Autodesk Inventor part; units mm, degrees
ref_plane "YZ Plane" through (0, 0, 0) normal (1, 0, 0) x (0, 1, 0)
ref_plane "XZ Plane" through (0, 0, 0) normal (0, 1, 0) x (-1, 0, 0)
ref_plane "XY Plane" through (0, 0, 0) normal (0, 0, 1) x (1, 0, 0)
sketch "スケッチ1" plane through (0, 0, 0) normal (0, 0, 1) x (1, 0, 0)
  line L0 (-4.5, 75) -> (4.5, 75)
  line L1 (4.5, 75) -> (4.5, -75)
  line L2 (4.5, -75) -> (-4.5, -75)
  line L3 (-4.5, -75) -> (-4.5, 75)
  line L4 (-4.5, 75) -> (4.5, -75) construction
  line L5 (4.5, 75) -> (-4.5, -75) construction
  circle A0 centre (0, 70) radius 1.7
  circle A1 centre (0, 50) radius 1.7
  circle A2 centre (0, 30) radius 1.7
  circle A3 centre (0, 10) radius 1.7
  circle A4 centre (0, -10) radius 1.7
  circle A5 centre (0, -30) radius 1.7
  circle A6 centre (0, -50) radius 1.7
  circle A7 centre (0, -70) radius 1.7
  point P0 (0, 0)
  dimension "d0" = 9
  dimension "d1" = 150
  dimension "d2" = 3.4
  dimension "d3" = 3.4
  dimension "d4" = 3.4
  dimension "d5" = 3.4
  dimension "d6" = 3.4
  dimension "d7" = 3.4
  dimension "d8" = 3.4
  dimension "d9" = 3.4
extrude "押し出し1" add sketch "スケッチ1" along normal blind 6.5
sketch "スケッチ2" plane through (0, 0, 6.5) normal (0, 0, 1) x (1, 0, 0)
  circle A0 centre (0, -70) radius 1.7
  circle A1 centre (0, -70) radius 2.9
  circle A2 centre (0, -50) radius 1.7
  circle A3 centre (0, -50) radius 2.9
  circle A4 centre (0, -30) radius 1.7
  circle A5 centre (0, -30) radius 2.9
  circle A6 centre (0, -10) radius 1.7
  circle A7 centre (0, -10) radius 2.9
  circle A8 centre (0, 10) radius 1.7
  circle A9 centre (0, 10) radius 2.9
  circle A10 centre (0, 30) radius 1.7
  circle A11 centre (0, 30) radius 2.9
  circle A12 centre (0, 50) radius 1.7
  circle A13 centre (0, 50) radius 2.9
  circle A14 centre (0, 70) radius 1.7
  circle A15 centre (0, 70) radius 2.9
  point P0 (0, 0)
  dimension "d12" = 5.8
  dimension "d13" = 5.8
  dimension "d14" = 5.8
  dimension "d15" = 5.8
  dimension "d16" = 5.8
  dimension "d17" = 5.8
  dimension "d18" = 5.8
  dimension "d19" = 5.8
extrude "押し出し2" cut sketch "スケッチ2" against normal blind 3.5
sketch "スケッチ3" plane through (-4.5, 75, 0) normal (0, 1, 0) x (1, 0, 0)
  line L0 (9, 0) -> (9, -6.5)
  line L1 (9, -4) -> (8, -4)
  line L2 (9, -4) -> (10, -4) construction
  line L3 (8, -4) -> (8, -4.7)
  line L4 (8, -4.7) -> (9, -4.7)
  line L5 (9, -4.7) -> (9, -4)
  line L6 (0, 0) -> (0, -6.5)
  line L7 (0, -4.7) -> (1, -4.7)
  line L8 (1, -4.7) -> (1, -4)
  line L9 (1, -4) -> (0, -4)
  line L10 (0, -4.7) -> (0, -4)
  point P0 (4.5, 0)
  dimension "d22" = 1
  dimension "d23" = 180
  dimension "d24" = 0.7
  dimension "d25" = 1
extrude "押し出し3" cut sketch "スケッチ3" against normal blind 150
chamfer "面取り1" distance 0.3 angle 45 4 edges at (4.5, 0, 4) (4.5, 0, 4.7) (-4.5, 0, 4) (-4.5, 0, 4.7)
chamfer "面取り2" distance 0.3 angle 45 8 edges at (-1.7, 70, 0) (-1.7, 50, 0) (-1.7, 30, 0) (-1.7, 10, 0) (-1.7, -10, 0) (-1.7, -30, 0) (-1.7, -50, 0) (-1.7, -70, 0)
properties part number "rail" material "鉄、可鍛鉄"
Input: part model. Units: mm. Frame: model coordinates. A direction names the side the tool comes from. Round coordinates to 2 decimals unless told otherwise and drop trailing zeros. Loops run counter-clockwise (first coordinate to the right, second up) from the corner with the lowest first, then second, coordinate; pieces in that order, holes last. Notation, with made-up numbers: (65.5, 85.5) -> (105.5, 85.5) arc R17 cw to (105.5, 94.5) -> close; hole circle Ø6 at (17, 70.5). An arc over 180 degrees is marked (long way). Answer as a JSON object with one key per item and string values. Group by question number.
1) Section query B-B on z = 2. State how many separate pieces and enclosed holes the cut face has, plus the area to 3 significant figures.
2) Reachability of faces 1 (the cylindrical face through (-0.37, -8.34, 1.63)), 2 (the flat face through (2, -50, 3)) from +Z, -Z, +X, -X, +Y, -Y: full face, straight path, thin tool, end or side. Return the list, or none.
3) Draft query along Y for faces 3 (the flat face through (4.5, 1, 2)), 4 (the flat face through (0, -12, 3)). Return one class per face: +Y half, -Y half, draft (parallel to the pull), parting line (faces both ways), or undercut.
4) Section query A-A on y = 70. Output: boundary loops of the cut face in (x, z), plus the area to 3 significant figures.
5) Ray query, L1, parallel to X at y = -70, z = 2.2; L2, parallel to X at y = 4.5, z = 4.25; L3, parallel to Z at x = 4, y = 63.5. Return the intervals inside material, ascending.
6) Pin query (flat end, axial travel): pin 1 (3.5 mm diameter, centred on x = 0, y = -10, fed in from -Z); pin 2 (1.7 mm diameter, centred on x = -0.5, y = -69, fed in from +Z). Return the tip coordinate at first contact, or that it passes through.
7) Section query C-C on y = 25. Output: boundary loops of the cut face in (x, z).
Reply:
{
 "1": {"separate pieces": "1", "enclosed holes": "8", "area": "1,280 mm2"},
 "2": {"face 1": "+Z, -Z", "face 2": "+Z"},
 "3": {"face 3": "draft", "face 4": "undercut"},
 "4": {"outline": "(-4.5, 0) -> (-2, 0) -> (-1.7, 0.3) -> (-1.7, 3) -> (-2.9, 3) -> (-2.9, 6.5) -> (-4.5, 6.5) -> (-4.5, 5) -> (-4.2, 4.7) -> (-3.5, 4.7) -> (-3.5, 4) -> (-4.2, 4) -> (-4.5, 3.7) -> close; (1.7, 0.3) -> (2, 0) -> (4.5, 0) -> (4.5, 3.7) -> (4.2, 4) -> (3.5, 4) -> (3.5, 4.7) -> (4.2, 4.7) -> (4.5, 5) -> (4.5, 6.5) -> (2.9, 6.5) -> (2.9, 3) -> (1.7, 3) -> close", "area": "26.3 mm2"},
 "5": {"L1": "x = -4.5 to -1.7, 1.7 to 4.5", "L2": "x = -3.5 to 3.5", "L3": "z = 0 to 4, 4.7 to 6.5"},
 "6": {"pin 1": "stops at z = 0.25", "pin 2": "stops at z = 3"},
 "7": {"outline": "(-4.5, 0) -> (4.5, 0) -> (4.5, 3.7) -> (4.2, 4) -> (3.5, 4) -> (3.5, 4.7) -> (4.2, 4.7) -> (4.5, 5) -> (4.5, 6.5) -> (-4.5, 6.5) -> (-4.5, 5) -> (-4.2, 4.7) -> (-3.5, 4.7) -> (-3.5, 4) -> (-4.2, 4) -> (-4.5, 3.7) -> close"}
}
